Check sheet for the modelled part. Datum: model origin and axes. Units: mm. Give positions to 0.01 mm unless a question says otherwise; leave off trailing zeros. Loops run counter-clockwise (first coordinate to the right, second up) from the corner with the lowest first, then second, coordinate; pieces in that order, holes last. Notation, with made-up numbers: M 63,-16 L 69,-16 A25 ccw 69,17 Z; hole C 29.5,61 d9. An arc over 180 degrees is marked long. Put each result on its own line as item: value. Start each with the question number.
Autodesk Inventor part; units mm, degrees
ref_plane "YZ Plane" through (0, 0, 0) normal (1, 0, 0) x (0, 1, 0)
ref_plane "XZ Plane" through (0, 0, 0) normal (0, 1, 0) x (-1, 0, 0)
ref_plane "XY Plane" through (0, 0, 0) normal (0, 0, 1) x (1, 0, 0)
sketch "Sketch1" plane through (0, 0, 0) normal (0, 0, 1) x (1, 0, 0)
  point P0 (0, 0)
sketch "Sketch2" plane through (0, 0, 0) normal (0, 0, 1) x (1, 0, 0)
  line L0 (-43, -31.5) -> (43, -31.5)
  line L1 (43, -31.5) -> (43, 31.5)
  line L2 (43, 31.5) -> (-43, 31.5)
  line L3 (-43, 31.5) -> (-43, -31.5)
  line L4 (-43, -31.5) -> (43, 31.5) construction
  line L5 (43, -31.5) -> (-43, 31.5) construction
  point P0 (0, 0)
  dimension "d0" = 86
  dimension "d1" = 63
extrude "Extrusion1" add sketch "Sketch2" along normal blind 3
sketch "Sketch3" plane through (0, 0, 3) normal (0, 0, 1) x (1, 0, 0)
  line L0 (-43, -31.5) -> (43, -31.5)
  line L1 (-43, -31.5) -> (-40, -31.5)
  line L2 (-40, -31.5) -> (-40, -1.5)
  line L3 (-40, -1.5) -> (-43, -1.5)
  line L4 (-43, -1.5) -> (-43, -31.5)
  line L5 (43, -31.5) -> (40, -31.5)
  line L6 (40, -31.5) -> (40, -1.5)
  line L7 (40, -1.5) -> (43, -1.5)
  line L8 (43, -1.5) -> (43, -31.5)
  line L9 (-40, -31.5) -> (-30, -31.5)
  line L10 (-30, -31.5) -> (-30, -28.5)
  line L11 (-30, -28.5) -> (-40, -28.5)
  line L12 (-40, -28.5) -> (-40, -31.5)
  line L13 (40, -31.5) -> (30, -31.5)
  line L14 (30, -31.5) -> (30, -28.5)
  line L15 (30, -28.5) -> (40, -28.5)
  line L16 (40, -28.5) -> (40, -31.5)
  line L17 (-10, -31.5) -> (10, -31.5)
  line L18 (10, -31.5) -> (10, -28.5)
  line L19 (10, -28.5) -> (-10, -28.5)
  line L20 (-10, -28.5) -> (-10, -31.5)
  line L21 (43, 31.5) -> (-43, 31.5)
  line L22 (-30, 31.5) -> (-10, 31.5)
  line L23 (-10, 31.5) -> (-10, 28.5)
  line L24 (-10, 28.5) -> (-30, 28.5)
  line L25 (-30, 28.5) -> (-30, 31.5)
  line L26 (10, 31.5) -> (30, 31.5)
  line L27 (30, 31.5) -> (30, 28.5)
  line L28 (30, 28.5) -> (10, 28.5)
  line L29 (10, 28.5) -> (10, 31.5)
  point P0 (0, 0)
  dimension "d4" = 3
  dimension "d5" = 3
  dimension "d6" = 10
  dimension "d7" = 3
  dimension "d8" = 10
  dimension "d9" = 3
  dimension "d10" = 20
  dimension "d11" = 3
  dimension "d12" = 20
  dimension "d13" = 3
  dimension "d16" = 30
extrude "Extrusion2" cut sketch "Sketch3" against normal through all
properties part number "cham_back"
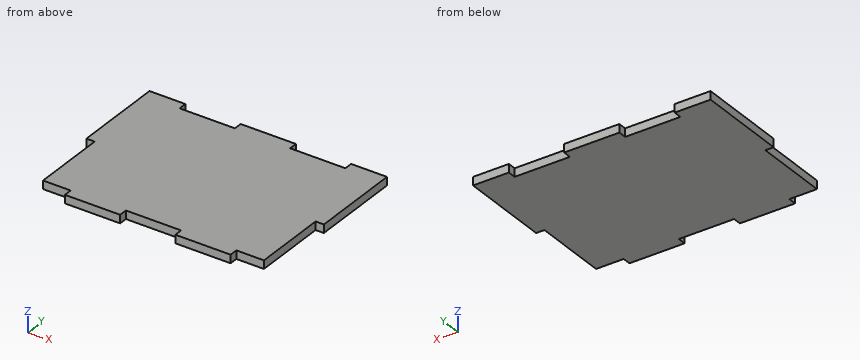
Q1. Section check B-B, the plane x = 15. Record the cut outline in (y, z).
Q2. Thickness scan on line 1 along Y through (x, z) = (0, 0.25); line 2 along X through (y, z) = (-24, 1); line 3 along Y through (x, z) = (-21, 1.4). Record the ranges inside material, lowest first. Write a range as [from, to].
Q3. Section check C-C, the plane y = -3. Record the cut outline in (x, z), then the cut area to 3 significant figures.
Q4. Section check A-A, the plane z = 1.3. Record the cut outline in (x, y), then the cut area to 3 significant figures.
Q5. Depth check by flat-ended pin: P1, Ø1.5, axis at x = -17, z = 1, coming from the +Y side; P2, Ø1.5, axis at y = -29.5, z = 1, coming from the -X side; P3, Ø0.9, axis at x = -36.5, z = 1.5, coming from the -Y side; P4, Ø12, axis at x = 29.5, y = -16, coming from the -Z side. Enter the tip coordinate at first touch or a pass-through.
Found:
1. outline: M -31.5,0 L 28.5,0 L 28.5,3 L -31.5,3 Z
2. line 1: y = [-28.5, 31.5]
2. line 2: x = [-40, 40]
2. line 3: y = [-31.5, 28.5]
3. outline: M -40,0 L 40,0 L 40,3 L -40,3 Z
3. area: 240 mm^2
4. outline: M -43,-1.5 L -40,-1.5 L -40,-28.5 L -30,-28.5 L -30,-31.5 L -10,-31.5 L -10,-28.5 L 10,-28.5 L 10,-31.5 L 30,-31.5 L 30,-28.5 L 40,-28.5 L 40,-1.5 L 43,-1.5 L 43,31.5 L 30,31.5 L 30,28.5 L 10,28.5 L 10,31.5 L -10,31.5 L -10,28.5 L -30,28.5 L -30,31.5 L -43,31.5 Z
4. area: 5,000 mm^2
5. P1: stops at y = 28.5
5. P2: stops at x = -30
5. P3: stops at y = -28.5
5. P4: stops at z = 0
